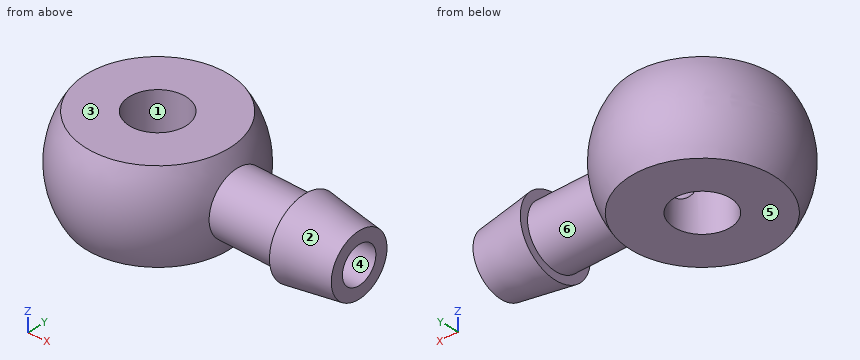
Autodesk Inventor part; units mm, degrees
ref_plane "YZ Plane" through (0, 0, 0) normal (1, 0, 0) x (0, 1, 0)
ref_plane "XZ Plane" through (0, 0, 0) normal (0, 1, 0) x (-1, 0, 0)
ref_plane "XY Plane" through (0, 0, 0) normal (0, 0, 1) x (1, 0, 0)
sketch "Sketch2" plane through (0, 0, 0) normal (0, 0, 1) x (1, 0, 0)
  circle A0 centre (0, 0) radius 4.7498
  line L0 (4.7498, 0) -> (-4.7498, 0)
  dimension "d1" = 4.7498
revolve "Revolution1" add sketch "Sketch2" angle 360 about axis through (4.7498, 0, 0) along (-1, 0, 0) picked at (-0.543, 3.0005) contours L0 A0
sketch "Sketch3" plane through (0, 0, 0) normal (0, 1, 0) x (-1, 0, 0)
  arc A0 (0, 4.7498) -> (0, -4.7498) centre (0, 0) ccw
  arc A1 (0, -4.7498) -> (0, 4.7498) centre (0, 0) ccw
  line L0 (-4.7498, 2.54) -> (4.7498, 2.54)
  line L1 (4.7498, 2.54) -> (4.7498, -2.54)
  line L2 (4.7498, -2.54) -> (-4.7498, -2.54)
  line L3 (-4.7498, -2.54) -> (-4.7498, 2.54)
  line L4 (0, 0) -> (0, 2.54)
  line L5 (-4.7498, 2.54) -> (4.7498, 2.54)
  line L6 (4.7498, 2.54) -> (4.7498, 4.7498)
  line L7 (4.7498, 4.7498) -> (-4.7498, 4.7498)
  line L8 (-4.7498, 4.7498) -> (-4.7498, 2.54)
  line L9 (-4.7498, -2.54) -> (4.7498, -2.54)
  line L10 (4.7498, -2.54) -> (4.7498, -4.7498)
  line L11 (4.7498, -4.7498) -> (-4.7498, -4.7498)
  line L12 (-4.7498, -4.7498) -> (-4.7498, -2.54)
  dimension "d3" = 5.08
  dimension "d5" = 2.54
extrude "Extrusion1" cut sketch "Sketch3" along normal mid plane 25.4 contours A1 L0 A0 | L7 L6 L0 A1 | A0 L0 L8 L7 | L2 A1 A0 | A0 L11 L12 L2 | L2 L10 L11 A1
sketch "Sketch5" plane through (0, 0, 0) normal (0, 1, 0) x (-1, 0, 0)
  line L0 (4.0136, -2.54) -> (-4.0136, -2.54)
  arc A0 (-4.0136, 2.54) -> (-4.0136, -2.54) centre (0, 0) ccw
  line L1 (-4.0136, 2.54) -> (4.0136, 2.54)
  arc A1 (4.0136, -2.54) -> (4.0136, 2.54) centre (0, 0) ccw
  line L2 (0, 0) -> (-18.5035, 0)
  line L3 (-11.2518, 0) -> (-11.2518, 1.7145)
  line L4 (-11.2518, 1.7145) -> (-8.2038, 2.159)
  line L5 (-8.2038, 2.159) -> (-8.2038, 1.7145)
  line L6 (-8.2038, 1.7145) -> (-4.4296, 1.7145)
  line L7 (-4.4296, 1.7145) -> (-4.4296, 0)
  line L8 (-11.2518, 0) -> (-4.4296, 0)
  dimension "d12" = 4.0136
  dimension "d15" = 3.429
  dimension "d16" = 4.318
  dimension "d17" = 15.2654
  dimension "d18" = 12.2174
revolve "Revolution2" add sketch "Sketch5" angle 360 about axis through (0, 0, 0) along (1, 0, 0) contours L2 L3 L4 L5 L6 A0 | A0 L7 L2
sketch "Sketch6" plane through (0, 0, 2.54) normal (0, 0, 1) x (1, 0, 0)
  circle A0 centre (0, 0) radius 4.0136
hole "Hole1" at (0, 0, 2.54) direction (0, 0, -1) diameter 3.175 end through all
sketch "Sketch7" plane through (11.2518, 0, 0) normal (1, 0, 0) x (0, 0, -1)
  circle A0 centre (0, 0) radius 1.7145
hole "Hole2" at (11.2518, 0, 0) direction (-1, 0, 0) diameter 2.0574 end up to surface
equation "\"d5\" = 0.5 * d3"
properties part number "Fuel Intake" material "Nylon, molybdenum disulphide"
Model file for the job. Use its own axes, mm. Face numbers are marked on the shaded views. A direction names the side the tool comes from. Coordinates: 2 decimals unless noted, no trailing zeros. Order: outer loops, then holes, each group sorted by start corner. A loop starts at its lowest first (then second) coordinate and runs counter-clockwise, first axis right, second up. Notation, with made-up numbers: (-1.5, -23) -> (46.5, -23) arc R16 cw to (46.5, -8) -> close; hole circle Ø9 at (88.5, 26). An arc over 180 degrees is marked (long way). Answer as a JSON object with one key per item and string values. Group by question number.
1) Which spindle directions (+Z, -Z, +X, -X, +Y, -Y) get a long thin tool onto all of the face, cutting with end or side? Do the marked faces 4, 5 and 6. Say none if no direction does.
2) Drill centre lines: L1, parallel to Y at x = 8, z = 0; L2, parallel to Z at x = 10.25, y = 0.5. Where is each one in solid material? Low to high.
3) Cut at C-C, the plane z = 0. Write the cut outline in (x, y) (1 decimal).
4) Flat gauge pins, fed straight in: pin 1 (1 mm diameter, centred on y = 3.5, z = 0, fed in from +X); pin 2 (3 mm diameter, centred on x = 9, z = 1.5, fed in from -Y); pin 3 (3 mm diameter, centred on x = 0, y = 0, fed in from -Z); pin 4 (3 mm diameter, centred on x = 3, z = 0, fed in from +Y). Where does each tip first touch, or does it go through?
5) Cut at D-D, the plane x = 7.5. Write the cut outline in (y, z), then the cut area to 3 significant figures.
6) Pull direction Y, two halves, no side cores. Call the marked faces 1, 2 and 3: +Y half, -Y half, draft (parallel to the pull), parting line (faces both ways), or undercut.
7) Cut at A-A, the plane x = 0. Write the cut outline in (y, z).
8) Cut at B-B, the plane y = 0. Write the cut outline in (x, z).
Check values:
{
 "1": {"face 4": "+X", "face 5": "-Z, +X, -X, +Y, -Y", "face 6": "none"},
 "2": {"L1": "y = -1.71 to -1.03, 1.03 to 1.71", "L2": "z = -1.79 to -0.9, 0.9 to 1.79"},
 "3": {"outline": "(1.2, -1) arc R1.6 cw (long way) to (1.2, 1) -> (11.3, 1) -> (11.3, 1.7) -> (8.2, 2.2) -> (8.2, 1.7) -> (4.4, 1.7) arc R4.7 ccw (long way) to (4.4, -1.7) -> (8.2, -1.7) -> (8.2, -2.2) -> (11.3, -1.7) -> (11.3, -1) -> close"},
 "4": {"pin 1": "stops at x = 3.68", "pin 2": "stops at y = -2.15", "pin 3": "passes through", "pin 4": "stops at y = 4.51"},
 "5": {"outline": "circle Ø3.43 at (0, 0); hole circle Ø2.06 at (0, 0)", "area": "5.91 mm²"},
 "6": {"face 1": "undercut", "face 2": "parting line", "face 3": "draft"},
 "7": {"outline": "(-4.01, -2.54) -> (-1.59, -2.54) -> (-1.59, 2.54) -> (-4.01, 2.54) arc R4.75 ccw to start; (1.59, -2.54) -> (4.01, -2.54) arc R4.75 ccw to (4.01, 2.54) -> (1.59, 2.54) -> close"},
 "8": {"outline": "(-4.01, -2.54) -> (-1.59, -2.54) -> (-1.59, 2.54) -> (-4.01, 2.54) arc R4.75 ccw to start; (1.59, -2.54) -> (4.01, -2.54) arc R4.75 ccw to (4.43, -1.71) -> (8.2, -1.71) -> (8.2, -2.16) -> (11.25, -1.71) -> (11.25, -1.03) -> (1.59, -1.03) -> close; (1.59, 1.03) -> (11.25, 1.03) -> (11.25, 1.71) -> (8.2, 2.16) -> (8.2, 1.71) -> (4.43, 1.71) arc R4.75 ccw to (4.01, 2.54) -> (1.59, 2.54) -> close"}
}
